from build123d import *

# Parameters (mm, degrees)
F0_W     = 275
F0_H     = 100
F1_DEPTH = 490
F3_DEPTH = 275.001
F5_DEPTH = 490.001


with BuildPart() as f1:
    # F0 (on Right) → F1 (new body)
    with BuildSketch(Plane.YZ):
        Rectangle(F0_W, F0_H)
    extrude(amount=F1_DEPTH)

    # F2 (on face) → F3 (cut, through all)
    with BuildSketch(Plane.XZ.offset(137.5)):
        Polygon((0, 50), (0, -50), (220, -50), align=None)
        Polygon((490, 50), (270, -50), (490, -50), align=None)
    extrude(amount=-F3_DEPTH, mode=Mode.SUBTRACT)

    # F4 (on Right) → F5 (cut, through all)
    with BuildSketch(Plane.YZ):
        Polygon((137.5, 50), (81.689713, -29.70535), (-137.5, 50), (-137.5, -50), (137.5, -50), align=None)
    extrude(amount=F5_DEPTH, mode=Mode.SUBTRACT)


solid = f1.part
CAD build for the part. Positions are in the model's coordinates, mm. Round coordinates to 2 decimals unless told otherwise and drop trailing zeros. Order: outer loops, then holes, each group sorted by start corner. A loop starts at its lowest first (then second) coordinate and runs counter-clockwise, first axis right, second up. Notation, with made-up numbers: M 35.25,54 L 77.25,54 A29 cw 77.25,82 Z; hole C -2,54 d7. An arc over 180 degrees is marked long. Use one line per item in the form item = value.
Q1. Saw through at A-A on x = 225. Give the cut face in (y, z), then the cut area to 3 significant figures.
Recorded:
outline = M -137.5,50 L 81.69,-29.71 L 137.5,50 Z
area = 11,000 mm^2
Q2. Saw through at B-B on z = 19.5. Give the cut face in (x, y) (3 decimals).
Recorded:
outline = M 67.1,-53.625 L 422.9,-53.625 L 422.9,116.144 L 67.1,116.144 Z
Q3. Probe L1, parallel to X at y = 30, z = 33; L2, parallel to X at y = 23, z = 41; L3, parallel to Z at x = 81, y = 94. List the from-to ranges inside material, lowest first.
Recorded:
L1 = 37.4 to 452.6
L2 = 19.8 to 470.2
L3 = 13.18 to 50
Q4. Saw through at C-C on y = 68. Give the cut face in (x, z).
Recorded:
outline = M 0,50 L 164.4,-24.73 L 325.6,-24.73 L 490,50 Z
Q5. Flat gauge pins, fed straight in: P1, Ø1, axis at y = 59.5, z = 11.5, coming from the -X side; P2, Ø3, axis at y = 75, z = -7.5, coming from the -X side; P3, Ø2, axis at x = 170, z = -0.5, coming from the +Y side. Where does each tip first touch, or does it go through?
Recorded:
P1 = 83.6
P2 = 123.2
P3 = 102.84
